Autodesk Inventor part; units mm, degrees
ref_plane "YZ Plane" through (0, 0, 0) normal (1, 0, 0) x (0, 1, 0)
ref_plane "XZ Plane" through (0, 0, 0) normal (0, 1, 0) x (-1, 0, 0)
ref_plane "XY Plane" through (0, 0, 0) normal (0, 0, 1) x (1, 0, 0)
sketch "Sketch1" plane through (0, 0, 0) normal (0, 0, 1) x (1, 0, 0)
  line L0 (0, 0) -> (150, 0)
  line L1 (150, 0) -> (150, -150)
  line L2 (150, -150) -> (0, -150)
  line L3 (0, -150) -> (0, 0)
  dimension "d0" = 150
  dimension "d1" = 150
extrude "Extrusion1" add sketch "Sketch1" along normal blind 20
sketch "Sketch2" plane through (0, 0, 20) normal (0, 0, 1) x (1, 0, 0)
  line L0 (24.5154, -22.5096) -> (124.5154, -22.5096)
  line L1 (124.5154, -22.5096) -> (124.5154, -122.5096)
  line L2 (124.5154, -122.5096) -> (24.5154, -122.5096)
  line L3 (24.5154, -122.5096) -> (24.5154, -22.5096)
  point P0 (0, 0)
  dimension "d4" = 100
  dimension "d5" = 100
extrude "Extrusion2" cut sketch "Sketch2" against normal blind 8
sketch "Sketch3" plane through (0, 0, 20) normal (0, 0, 1) x (1, 0, 0)
  point P0 (0, 0)
  point P1 (10.7394, -12.154)
  point P2 (136.4315, -10.9415)
  point P3 (137.6439, -139.4626)
  point P4 (11.1436, -137.846)
hole "Hole1" at (10.7394, -12.154, 20) at (136.4315, -10.9415, 20) at (137.6439, -139.4626, 20) at (11.1436, -137.846, 20) direction (0, 0, -1) diameter 10 depth 30 tip angle 118
properties part number "carromboard15cm"
Input: part model. Units: mm. Frame: model coordinates. A direction names the side the tool comes from. Coordinates: 2 decimals unless noted, no trailing zeros. Loops run counter-clockwise (first coordinate to the right, second up) from the corner with the lowest first, then second, coordinate; pieces in that order, holes last. Notation, with made-up numbers: (-23, 75.5) -> (-1, 75.5) arc R15 cw to (-1, 94.5) -> close; hole circle Ø5 at (0.25, -22). An arc over 180 degrees is marked (long way). Write item = value, one per line. Start each with the question number.
Item 1: Reachability of faces 1 (the face through (24.515, -73, 16)), 2 (the face through (141.313, -9.858, 9.86)) from +Z, -Z, +X, -X, +Y, -Y: full face, straight path, thin tool, end or side. Return the list, or none.
Item 2: Cut plane C-C, the plane z = 17.75. Return loops of the section in (x, y).
Item 3: Cut plane A-A, the plane x = 35. Return loops of the section in (y, z), plus the area to 3 significant figures.
Item 4: First-contact query: P1, Ø2, axis at x = 103, y = -43, coming from the +Z side. Flat tip, straight axial feed; report the tip coordinate or a pass-through.
Item 5: Mould query, pull axis Y, two halves, no side actions, for faces 3 (the face through (0, -76, 10)), 4 (the face through (74, 0, 10)), 5 (the face through (124.515, -72, 16)). Classes: pulls with the +Y half, pulls with the -Y half, needs draft (parallel to the pull), parting line crosses it, or undercut.
Item 6: Cut plane D-D, the plane y = -10.5. Return loops of the section in (x, z), plus the area to 3 significant figures.
Item 7: Cut plane B-B, the plane y = -26. Return loops of the section in (x, z), plus the area to 3 significant figures.
Item 8: Material intervals for line 1 (Y direction, x = 42.5, z = 17.5); line 2 (Y direction, x = 12, z = 8.75); line 3 (X direction, y = -114, z = 19.25), sorted ascending.
Ans:
q1.face_1 = +Z
q1.face_2 = +Z, -Z
q2.outline = (0, -150) -> (150, -150) -> (150, 0) -> (0, 0) -> close; hole circle Ø10 at (10.74, -12.15); hole circle Ø10 at (11.14, -137.85); hole (24.52, -122.51) -> (124.52, -122.51) -> (124.52, -22.51) -> (24.52, -22.51) -> close; hole circle Ø10 at (136.43, -10.94); hole circle Ø10 at (137.64, -139.46)
q3.outline = (-150, 0) -> (0, 0) -> (0, 20) -> (-22.51, 20) -> (-22.51, 12) -> (-122.51, 12) -> (-122.51, 20) -> (-150, 20) -> close
q3.area = 2,200 mm²
q4.P1 = 12
q5.face_3 = needs draft
q5.face_4 = pulls with the +Y half
q5.face_5 = undercut
q6.outline = (0, 0) -> (6.02, 0) -> (6.02, 20) -> (0, 20) -> close; (15.46, 0) -> (131.45, 0) -> (131.45, 20) -> (15.46, 20) -> close; (141.41, 0) -> (150, 0) -> (150, 20) -> (141.41, 20) -> close
q6.area = 2,610 mm²
q7.outline = (0, 0) -> (150, 0) -> (150, 20) -> (124.52, 20) -> (124.52, 12) -> (24.52, 12) -> (24.52, 20) -> (0, 20) -> close
q7.area = 2,200 mm²
q8.line_1 = -150 to -122.51, -22.51 to 0
q8.line_2 = -150 to -142.77, -132.92 to -16.99, -7.32 to 0
q8.line_3 = 0 to 24.52, 124.52 to 150
